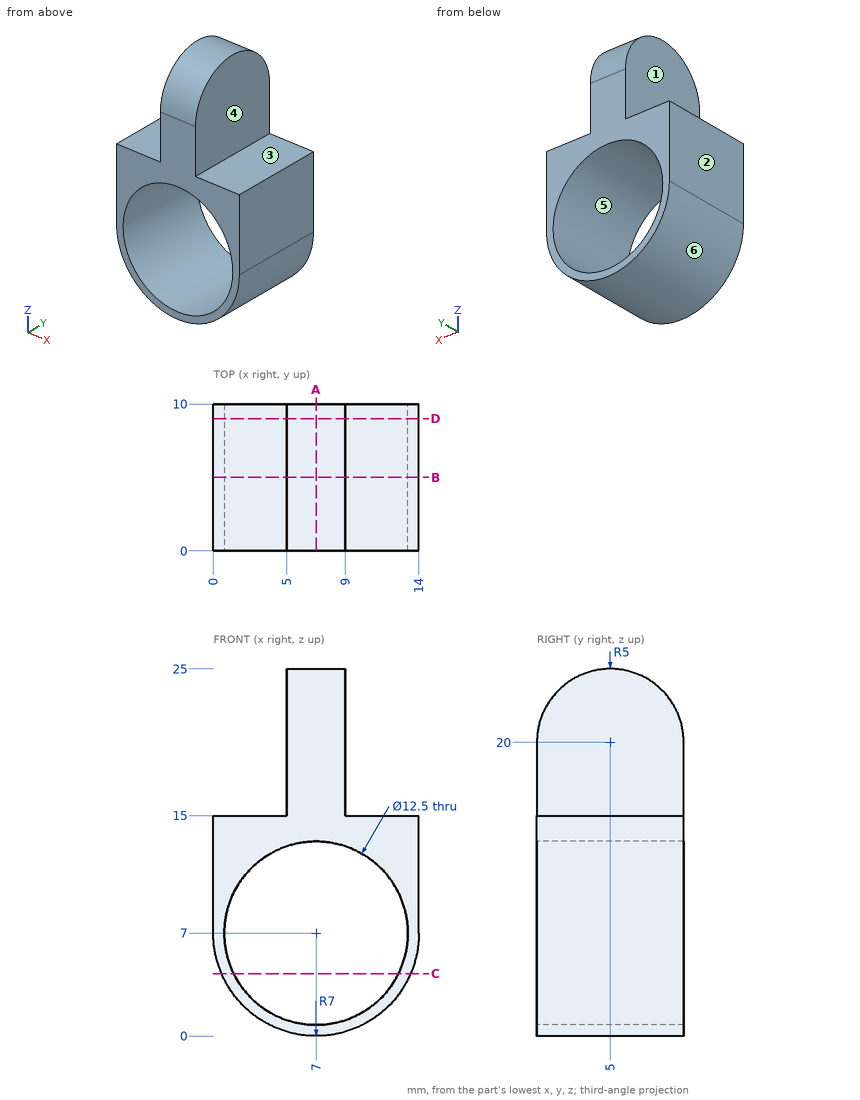
Drawing for the job (mm, zero at the part's lowest x, y, z). A direction names the side the tool comes from. Round coordinates to 2 decimals unless told otherwise and drop trailing zeros. Order: outer loops, then holes, each group sorted by start corner. A loop starts at its lowest first (then second) coordinate and runs counter-clockwise, first axis right, second up.
Item 1: Mould opens along Z. For the marked faces 4, 5 and 6 say: pulls with the +Z half, pulls with the -Z half, needs draft (parallel to the pull), parting line crosses it, or undercut.
Item 2: Saw through at D-D on y = 9. Write the cut outline in (x, z).
Item 3: Probe line 1 along X through (y, z) = (3.5, 7); line 2 along X through (y, z) = (3, 17); line 3 along Z through (x, y) = (9.5, 7.75). List the from-to ranges inside material, lowest first.
Item 4: Saw through at B-B on y = 5. Write the cut outline in (x, z).
Item 5: Pin check, flat tips, straight feed: pin 1 (4 mm diameter, centred on x = 11.5, y = 2.5, fed in from +Z); pin 2 (5 mm diameter, centred on x = 8.5, y = 2, fed in from +Z); pin 3 (3 mm diameter, centred on y = 4, z = 21.5, fed in from +X). Stop position of each tip, or through.
Item 6: Saw through at A-A on x = 7. Write the cut outline in (y, z), then the cut area to 3 significant figures.
Item 7: Tool access for the marked faces 1, 2 and 3: list every direction of +Z, -Z, +X, -X, +Y, -Y with a clear straight run to the whole face (end or side of a thin tool).
Item 8: Saw through at C-C on z = 4.25. Write the cut outline in (x, y), then the cut area to 3 significant figures.
Reported:
1. face 4: needs draft
1. face 5: undercut
1. face 6: pulls with the -Z half
2. outline: (0, 7) arc R7 ccw to (14, 7) - (14, 15) - (9, 15) - (9, 23) - (5, 23) - (5, 15) - (0, 15) - close; hole circle Ø12.5 at (7, 7)
3. line 1: x = 0 to 0.75, 13.25 to 14
3. line 2: x = 5 to 9
3. line 3: z = 0.46 to 1.27, 12.73 to 15
4. outline: (0, 7) arc R7 ccw to (14, 7) - (14, 15) - (9, 15) - (9, 25) - (5, 25) - (5, 15) - (0, 15) - close; hole circle Ø12.5 at (7, 7)
5. pin 1: stops at z = 15
5. pin 2: stops at z = 24.97
5. pin 3: stops at x = 9
6. outline: (0, 0) - (10, 0) - (10, 0.75) - (0, 0.75) - close; (0, 13.25) - (10, 13.25) - (10, 20) arc R5 ccw to (0, 20) - close
6. area: 114 mm2
7. face 1: +Z, -X, +Y, -Y
7. face 2: +Z, -Z, -X, +Y, -Y
7. face 3: +Z, +X, +Y, -Y
8. outline: (0.56, 0) - (1.39, 0) - (1.39, 10) - (0.56, 10) - close; (12.61, 0) - (13.44, 0) - (13.44, 10) - (12.61, 10) - close
8. area: 16.5 mm2
